```python
from build123d import *

# Parameters (mm, degrees)
SKETCH1_R           = 4.25
BOSS_EXTRUDE1_DEPTH = 0.5
FILLET1_R           = 0.508
SKETCH2_R           = 1.25
BOSS_EXTRUDE2_DEPTH = 1.75
SKETCH3_R           = 1.5
BOSS_EXTRUDE3_DEPTH = 1.75
FILLET2_R           = 1.27


with BuildPart() as part:
    # Sketch1 → Boss-Extrude1 (new body)
    with BuildSketch(Plane.XY):
        Circle(SKETCH1_R)
    extrude(amount=BOSS_EXTRUDE1_DEPTH)

    # Fillet1
    # the kernel refuses this fillet: 0.508 mm, written as the material it takes off along each edge
    with BuildSketch(Plane(origin=(0, 0, 0), x_dir=(1, 0, 0), z_dir=(0, -1, 0))) as fillet1_piece_1:
        with BuildLine():
            CenterArc((4.25 - FILLET1_R, FILLET1_R), FILLET1_R, 270, 90)
            Line((4.25 - FILLET1_R, 0), (4.25, 0))
            Line((4.25, 0), (4.25, FILLET1_R))
        make_face()
    revolve(axis=Axis((0, 0, 0), (0, 0, 1)), mode=Mode.SUBTRACT)

    # Sketch2 → Boss-Extrude2 (add)
    with BuildSketch(Plane.XY.offset(0.5)):
        Circle(SKETCH2_R)
    extrude(amount=BOSS_EXTRUDE2_DEPTH)

    # Sketch3 → Boss-Extrude3 (add)
    with BuildSketch(Plane.XY.offset(2.25)):
        Circle(SKETCH3_R)
    extrude(amount=BOSS_EXTRUDE3_DEPTH)

    # Fillet2
    fillet2_edges = [part.edges().sort_by_distance(p)[0] for p in [
        (-1.5, 0, 4),
    ]]
    fillet(fillet2_edges, radius=FILLET2_R)


solid = part.part
```
Design review of the part built by this model. Coordinates are the model's own, in mm. Coordinates: 2 decimals unless noted, no trailing zeros. Write each loop counter-clockwise with the first axis right and the second up, starting at its lowest first coordinate (ties: lowest second). Pieces come first, ordered by that corner, then holes.
1) Mouldability with a two-part tool opening along Z and no side actions: class faces 1 (the flat face through (0, 0, 0)), 2 (the cylindrical face through (-0.27, -1.22, 1.36)), 3 (the cylindrical face through (-1.5, 0.07, 2.49)) as +Z half, -Z half, draft (parallel to the pull), parting line (faces both ways), or undercut.
2) Add section A-A (z = 2.5). Write out the cut boundary in (x, y).
3) To check wall thickness, follow L1, parallel to Y at x = 0, z = 0.9; L2, parallel to Z at x = 0, y = 3.75; L3, parallel to Z at x = -1, y = -4. State the ranges of each line that lie inside material, in increasing order.
4) Add section B-B (z = 0.8). Write out the cut boundary in (x, y), plus the area to 3 significant figures.
5) Insertion check: pin 1 (1.5 mm diameter, centred on x = 0.5, y = 0, fed in from -Z); pin 2 (2 mm diameter, centred on x = 0, y = 3, fed in from +Z); pin 3 (2 mm diameter, centred on y = -1, z = 3.5, fed in from -X). Each pin has a flat end and moves straight along its axis. Give the tip position at first contact, or say it passes through.
Check result:
1. face 1: -Z half
1. face 2: undercut
1. face 3: draft
2. outline: circle Ø3 at (0, 0)
3. L1: y = -1.25 to 1.25
3. L2: z = 0 to 0.5
3. L3: z = 0.17 to 0.5
4. outline: circle Ø2.5 at (0, 0)
4. area: 4.91 mm2
5. pin 1: stops at z = 0
5. pin 2: stops at z = 0.5
5. pin 3: stops at x = -1.48
